from build123d import *

# Parameters (mm, degrees)
F1_DEPTH = 12.7
F2_R     = 6.669357
F3_DEPTH = 45.974


with BuildPart() as f1:
    # F0 (on Front) → F1 (new body)
    with BuildSketch(Plane.XZ):
        Polygon((-10.710431, 18.454035), (-21.336878, -0.048488), (-10.626448, -18.502522), (10.710431, -18.454035), (21.336878, 0.048488), (10.626448, 18.502522), align=None)
    extrude(amount=-F1_DEPTH)

    # F2 (on face) → F3 (join)
    with BuildSketch(Plane.XZ):
        Circle(F2_R)
    extrude(amount=F3_DEPTH)


solid = f1.part
Can you work these out from the model? Positions are in its coordinate system, mm. A direction names the side the tool comes from. Round coordinates to 2 decimals unless told otherwise and drop trailing zeros. Write each loop counter-clockwise with the first axis right and the second up, starting at its lowest first coordinate (ties: lowest second). Pieces come first, ordered by that corner, then holes. Notation, with made-up numbers: (11, 28) -> (45, 28) arc R26 ccw to (45, 63) -> close; hole circle Ø4 at (4.25, 16). An arc over 180 degrees is marked (long way). Use one line per item in the form item = value. Start each with the question number.
Q1. Imagine slicing it at B-B (x = 1.5). Please give me the cut outline in (y, z).
Q2. If I drill on probe 1 along Y at (x, z) = (14, -11); probe 2 along Z at (x, y) = (4.5, 4); probe 3 along Z at (x, y) = (-1.5, -5), over which ranges is the centre line in solid material (lowest first)? Write a range as [from, to].
Q3. Imagine slicing it at D-D (y = -3). Please give me the cut outline in (x, z).
Q4. I'm going to push flat-ended pins straight in: P1, Ø12, axis at y = -15.5, z = 9, coming from the -X side; P2, Ø2, axis at y = -31.5, z = 0.5, coming from the +X side; P3, Ø1.5, axis at x = -4, y = -27.5, coming from the +Z side. Where does each tip first touch, or does it pass through?
Q5. Imagine slicing it at C-C (z = 11). Please give me the cut outline in (x, y), then the cut area to 3 significant figures.
Q6. Which directions (+Z, -Z, +X, -X, +Y, -Y) give clear straight access to the entire face, cutting with the end or side of a thin tool? Please do faces 1 (the face through (-15.95, 6.26, 9.33)), 2 (the face through (6.361, -22.665, 2.003)).
Q7. Imagine slicing it at A-A (y = 6.5). Please give me the cut outline in (x, z), then the cut area to 3 significant figures.
Worked out:
q1.outline = (-45.97, -6.5) -> (0, -6.5) -> (0, -18.47) -> (12.7, -18.47) -> (12.7, 18.48) -> (0, 18.48) -> (0, 6.5) -> (-45.97, 6.5) -> close
q2.probe_1 = [0, 12.7]
q2.probe_2 = [-18.47, 18.49]
q2.probe_3 = [-6.5, 6.5]
q3.outline = circle Ø13.34 at (0, 0)
q4.P1 = -5.96
q4.P2 = 6.67
q4.P3 = 5.82
q5.outline = (-14.99, 0) -> (14.98, 0) -> (14.98, 12.7) -> (-14.99, 12.7) -> close
q5.area = 381 mm^2
q6.face_1 = +Z, -X, +Y, -Y
q6.face_2 = -Y
q7.outline = (-21.34, -0.05) -> (-10.63, -18.5) -> (10.71, -18.45) -> (21.34, 0.05) -> (10.63, 18.5) -> (-10.71, 18.45) -> close
q7.area = 1,180 mm^2
